Geometry: final body of the model. Coordinates: model frame, mm. A direction names the side the tool comes from. Give positions to 0.01 mm unless a question says otherwise; leave off trailing zeros. Order: outer loops, then holes, each group sorted by start corner. A loop starts at its lowest first (then second) coordinate and runs counter-clockwise, first axis right, second up. Notation, with made-up numbers: (39.5, -29) -> (90.5, -29) arc R21 cw to (90.5, -9) -> close; hole circle Ø4 at (40.25, 69.25). An arc over 180 degrees is marked (long way). One line per question, with ' | ' between items. Start each with the question number.
(1) Ray query, L1, parallel to Z at x = -2, y = 1.5; L2, parallel to Z at x = 6.5, y = 2.55; L3, parallel to X at y = 1.8, z = -1. Return the intervals inside material, ascending.
(2) Set-up query: faces 1 (the face through (2.9, 1, 0)), 2 (the face through (0, 1, -1.7)), 3 (the face through (-2.9, 1, -12)), 4 (the face through (0, 0, 0)). Return all of +Z, -Z, +X, -X, +Y, -Y with unobstructed straight access to the full face (end or side cutting, diameter ignored); none if empty.
(3) Section A-A (z = -7.75). Return loops of the section in (x, y), then the cut area to 3 significant figures.
(4) Mould query, pull axis Z, two halves, no side actions, for faces 5 (the face through (9, 2.4, -13)), 6 (the face through (0, 1, -13.349)), 7 (the face through (0, 1, -7.529)), 8 (the face through (0, 1, 1.7)). Classes: +Z half, -Z half, draft (parallel to the pull), parting line (faces both ways), or undercut.
(5) Section C-C (x = 7.75). Return loops of the section in (y, z), then the cut area to 3 significant figures.
(6) Section B-B (y = 0.9). Return loops of the section in (x, z).
(7) First-contact query: pin 1 Ø0.7 at (x, y) = (5.5, 3) entering from -Z; pin 2 Ø1.6 at (y, z) = (1.5, -11.5) entering from -X; pin 3 Ø1.6 at (y, z) = (1, -6) entering from +X. Flat tips, straight axial feed; report the tip coordinate or a pass-through.
(8) Section D-D (z = -6). Return loops of the section in (x, y), then the cut area to 3 significant figures.
```python
from build123d import *

# Parameters (mm, degrees)
EXTRUDE_1_DEPTH     = 3
EXTRUDE_1_2_DEPTH   = 3
EXTRUDE_1_3_DEPTH   = 3
SKETCH_2_W          = 7
SKETCH_2_H          = 5
EXTRUDE_2_DEPTH     = 0.6
SKETCH_3_W          = 6
SKETCH_3_H          = 1.2
EXTRUDE_3_DEPTH     = 0.6
SKETCH_4_W          = 1
SKETCH_4_H          = 13
EXTRUDE_4_DEPTH     = 0.6
FILLET_1_R          = 0.5
SKETCH_5_W          = 1
SKETCH_5_H          = 0.6
EXTRUDE_5_DEPTH     = 1.2
CUT_EXTRUDE_1_DEPTH = 1


with BuildPart() as part:
    # Sketch 1 → Extrude 1 (new body)
    with BuildSketch(Plane(origin=(0, 0, 0), x_dir=(1, 0, 0), z_dir=(0, 1, 0))):
        with BuildLine():
            Line((-2.2, 1.7), (2.2, 1.7))
            ThreePointArc((2.2, 1.7), (2.694974747, 1.494974747), (2.9, 1))
            Line((2.9, 1), (2.9, -1))
            ThreePointArc((2.9, -1), (2.694974747, -1.494974747), (2.2, -1.7))
            Line((2.2, -1.7), (-2.2, -1.7))
            ThreePointArc((-2.2, -1.7), (-2.694974747, -1.494974747), (-2.9, -1))
            Line((-2.9, -1), (-2.9, 1))
            ThreePointArc((-2.9, 1), (-2.694974747, 1.494974747), (-2.2, 1.7))
        make_face()
    extrude(amount=EXTRUDE_1_DEPTH)



with BuildPart() as body_2:
    # Sketch 1 → Extrude 1 2 (new body)
    with BuildSketch(Plane(origin=(0, 0, 0), x_dir=(1, 0, 0), z_dir=(0, 1, 0))):
        with BuildLine():
            Line((-2.2, 7.528722779), (2.2, 7.528722779))
            ThreePointArc((2.2, 7.528722779), (2.694974747, 7.323697526), (2.9, 6.828722779))
            Line((2.9, 6.828722779), (2.9, 4.828722779))
            ThreePointArc((2.9, 4.828722779), (2.694974747, 4.333748032), (2.2, 4.128722779))
            Line((2.2, 4.128722779), (-2.2, 4.128722779))
            ThreePointArc((-2.2, 4.128722779), (-2.694974747, 4.333748032), (-2.9, 4.828722779))
            Line((-2.9, 4.828722779), (-2.9, 6.828722779))
            ThreePointArc((-2.9, 6.828722779), (-2.694974747, 7.323697526), (-2.2, 7.528722779))
        make_face()
    extrude(amount=EXTRUDE_1_2_DEPTH)


with BuildPart() as body_3:
    # Sketch 1 → Extrude 1 3 (new body)
    with BuildSketch(Plane(origin=(0, 0, 0), x_dir=(1, 0, 0), z_dir=(0, 1, 0))):
        with BuildLine():
            Line((-2.2, 13.349128593), (2.2, 13.349128593))
            ThreePointArc((2.2, 13.349128593), (2.694974747, 13.144103339), (2.9, 12.649128593))
            Line((2.9, 12.649128593), (2.9, 10.649128593))
            ThreePointArc((2.9, 10.649128593), (2.694974747, 10.154153846), (2.2, 9.949128593))
            Line((2.2, 9.949128593), (-2.2, 9.949128593))
            ThreePointArc((-2.2, 9.949128593), (-2.694974747, 10.154153846), (-2.9, 10.649128593))
            Line((-2.9, 10.649128593), (-2.9, 12.649128593))
            ThreePointArc((-2.9, 12.649128593), (-2.694974747, 13.144103339), (-2.2, 13.349128593))
        make_face()
    extrude(amount=EXTRUDE_1_3_DEPTH)


with BuildPart() as part_1:
    add(part.part)

    add(body_2.part)  # Extrude 2 merges body 2

    add(body_3.part)  # Extrude 2 merges body 3
    # Sketch 2 → Extrude 2 (add)
    with BuildSketch(Plane(origin=(0, 3, 0), x_dir=(1, 0, 0), z_dir=(0, 1, 0))):
        with Locations((0.036699987, 11.763062551)):
            Rectangle(SKETCH_2_W, SKETCH_2_H)
        with Locations((0.036699987, 5.863062551)):
            Rectangle(SKETCH_2_W, SKETCH_2_H)
        with Locations((0.036699987, -0.036937449)):
            Rectangle(SKETCH_2_W, SKETCH_2_H)
    extrude(amount=-EXTRUDE_2_DEPTH)

    # Sketch 3 → Extrude 3 (add)
    with BuildSketch(Plane(origin=(0, 3, 0), x_dir=(1, 0, 0), z_dir=(0, 1, 0))):
        with Locations((6.536699987, 11.763062551)):
            Rectangle(SKETCH_3_W, SKETCH_3_H)
        with Locations((6.536699987, 5.863062551)):
            Rectangle(SKETCH_3_W, SKETCH_3_H)
        with Locations((6.536699987, -0.036937449)):
            Rectangle(SKETCH_3_W, SKETCH_3_H)
    extrude(amount=-EXTRUDE_3_DEPTH)

    # Sketch 4 → Extrude 4 (add)
    with BuildSketch(Plane.XZ.offset(-2.4)):
        with Locations((9.036699987, -5.863062551)):
            Rectangle(SKETCH_4_W, SKETCH_4_H)
    extrude(amount=-EXTRUDE_4_DEPTH)

    # Fillet 1
    fillet_1_edges = [part_1.edges().sort_by_distance(p)[0] for p in [
        (3.536699987, 2.7, -11.163062551),
        (3.536699987, 2.7, -12.363062551),
        (3.536699987, 2.7, 0.636937449),
        (3.536699987, 2.7, -0.563062551),
        (3.536699987, 2.7, -5.263062551),
        (3.536699987, 2.7, -6.463062551),
    ]]
    fillet(fillet_1_edges, radius=FILLET_1_R)

    # Sketch 5 → Extrude 5 (add)
    with BuildSketch(Plane(origin=(0, 0, -12.363062551), x_dir=(-1, 0, 0), z_dir=(0, 0, -1))):
        with Locations((-9.036699987, 2.7)):
            Rectangle(SKETCH_5_W, SKETCH_5_H)
    extrude(amount=EXTRUDE_5_DEPTH)

    # Sketch 6 → Cut-Extrude 1 (cut)
    with BuildSketch(Plane.ZY.offset(-8.536699987)):
        Polygon((-12.363062551, 2.4), (-12.363062551, 2.7), (-12.720178884, 2.4), align=None)
    extrude(amount=-CUT_EXTRUDE_1_DEPTH, mode=Mode.SUBTRACT)


solid = part_1.part
```
Response:
1) L1: z = -13.35 to -9.95, -7.53 to -4.13, -1.7 to 1.7 | L2: z = -12.36 to -11.16, -6.46 to -5.26, -0.56 to 0.64 | L3: x = -2.9 to 2.9
2) face 1: +Z, -Z, +X, -Y | face 2: +X, -X, -Y | face 3: +Z, -Z, -X, -Y | face 4: +Z, -Z, +X, -X, -Y
3) outline: (-3.46, 2.4) -> (3.54, 2.4) -> (3.54, 3) -> (-3.46, 3) -> close; (8.54, 2.4) -> (9.54, 2.4) -> (9.54, 3) -> (8.54, 3) -> close | area: 4.80 mm^2
4) face 5: draft | face 6: -Z half | face 7: undercut | face 8: +Z half
5) outline: (2.4, -12.36) -> (3, -12.36) -> (3, -11.16) -> (2.4, -11.16) -> close; (2.4, -6.46) -> (3, -6.46) -> (3, -5.26) -> (2.4, -5.26) -> close; (2.4, -0.56) -> (3, -0.56) -> (3, 0.64) -> (2.4, 0.64) -> close | area: 2.16 mm^2
6) outline: (-2.9, -12.65) arc R0.7 ccw to (-2.2, -13.35) -> (2.2, -13.35) arc R0.7 ccw to (2.9, -12.65) -> (2.9, -10.65) arc R0.7 ccw to (2.2, -9.95) -> (-2.2, -9.95) arc R0.7 ccw to (-2.9, -10.65) -> close; (-2.9, -6.83) arc R0.7 ccw to (-2.2, -7.53) -> (2.2, -7.53) arc R0.7 ccw to (2.9, -6.83) -> (2.9, -4.83) arc R0.7 ccw to (2.2, -4.13) -> (-2.2, -4.13) arc R0.7 ccw to (-2.9, -4.83) -> close; (-2.9, -1) arc R0.7 ccw to (-2.2, -1.7) -> (2.2, -1.7) arc R0.7 ccw to (2.9, -1) -> (2.9, 1) arc R0.7 ccw to (2.2, 1.7) -> (-2.2, 1.7) arc R0.7 ccw to (-2.9, 1) -> close
7) pin 1: stops at z = -12.36 | pin 2: stops at x = -2.9 | pin 3: stops at x = 2.9
8) outline: (-3.46, 2.4) -> (-2.9, 2.4) -> (-2.9, 0) -> (2.9, 0) -> (2.9, 2.4) -> (9.54, 2.4) -> (9.54, 3) -> (-3.46, 3) -> close | area: 21.7 mm^2
